Build history of the part. All positions in model axes, mm. Face numbers are marked on the shaded views. A direction names the side the tool comes from. Give positions to 0.01 mm unless a question says otherwise; leave off trailing zeros. Write each loop counter-clockwise with the first axis right and the second up, starting at its lowest first coordinate (ties: lowest second). Pieces come first, ordered by that corner, then holes. Notation, with made-up numbers: M -9,6.25 L 24,6.25 A26 ccw 24,26.25 Z; hole C 62,14.25 d11. An arc over 180 degrees is marked long. Return JSON: item names as keys, results as strings. Group by question number.
Q1. Band-saw the part on C-C, the plane x = -4. Give the cut face in (y, z), then the cut area to 3 significant figures.
Q2. Band-saw the part on D-D, the plane x = 26.5. Give the cut face in (y, z), then the cut area to 3 significant figures.
Q3. Band-saw the part on A-A, the plane y = 0. Give the cut face in (x, z), then the cut area to 3 significant figures.
Q4. Flat gauge pins, fed straight in: pin 1 Ø4 at (x, y) = (61.5, 6) entering from +Z; pin 2 Ø5 at (x, z) = (85.5, 10) entering from +Y; pin 3 Ø2 at (x, z) = (17.5, 12.5) entering from +Y. Where does each tip first touch, or does it go through?
Q5. Wall check: probe 1 along X at (y, z) = (16, -8); probe 2 along Z at (x, y) = (38, 10); probe 3 along Z at (x, y) = (3, -6). Give the ranges that are in metal, low to high.
Q6. Tool access for the marked faces 1 and 2: list every direction of +Z, -Z, +X, -X, +Y, -Y with a clear straight run to the whole face (end or side of a thin tool).
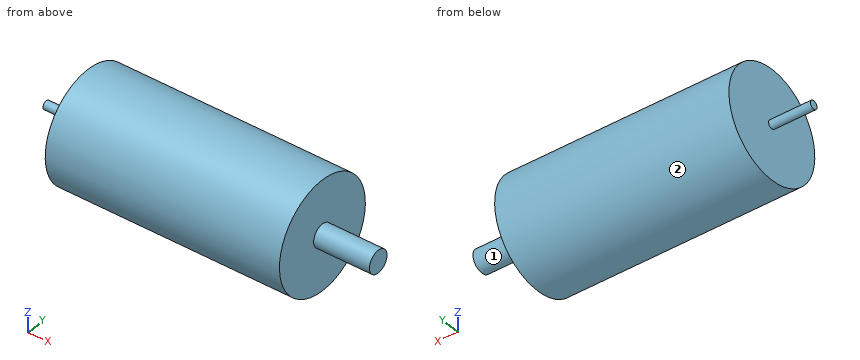
from build123d import *

# Parameters (mm, degrees)
SKETCH1_R           = 19.5
BOSS_EXTRUDE1_DEPTH = 84
SKETCH2_R           = 4
BOSS_EXTRUDE2_DEPTH = 20
SKETCH3_R           = 1.5
BOSS_EXTRUDE3_DEPTH = 15


with BuildPart() as part:
    # Sketch1 → Boss-Extrude1 (new body)
    with BuildSketch(Plane(origin=(0, 0, 0), x_dir=(0, 0, -1), z_dir=(1, 0, 0))):
        Circle(SKETCH1_R)
    extrude(amount=BOSS_EXTRUDE1_DEPTH)

    # Sketch2 → Boss-Extrude2 (add)
    with BuildSketch(Plane(origin=(84, 0, 0), x_dir=(0, 0, -1), z_dir=(1, 0, 0))):
        Circle(SKETCH2_R)
    extrude(amount=BOSS_EXTRUDE2_DEPTH)

    # Sketch3 → Boss-Extrude3 (add)
    with BuildSketch(Plane.ZY):
        Circle(SKETCH3_R)
    extrude(amount=BOSS_EXTRUDE3_DEPTH)


solid = part.part
From the geometry:
{
 "1": {"outline": "C 0,0 d3", "area": "7.07 mm^2"},
 "2": {"outline": "C 0,0 d39", "area": "1,190 mm^2"},
 "3": {"outline": "M -15,-1.5 L 0,-1.5 L 0,-19.5 L 84,-19.5 L 84,-4 L 104,-4 L 104,4 L 84,4 L 84,19.5 L 0,19.5 L 0,1.5 L -15,1.5 Z", "area": "3,480 mm^2"},
 "4": {"pin 1": "stops at z = 19.09", "pin 2": "stops at y = 17.78", "pin 3": "stops at y = 15.75"},
 "5": {"probe 1": "x = 0 to 84", "probe 2": "z = -16.74 to 16.74", "probe 3": "z = -18.55 to 18.55"},
 "6": {"face 1": "+X", "face 2": "+X, -X"}
}
